Read the model definition and answer for the solid it produces. Units are mm, in the model's axes. Coordinates: 2 decimals unless noted, no trailing zeros. Order: outer loops, then holes, each group sorted by start corner. A loop starts at its lowest first (then second) coordinate and runs counter-clockwise, first axis right, second up.
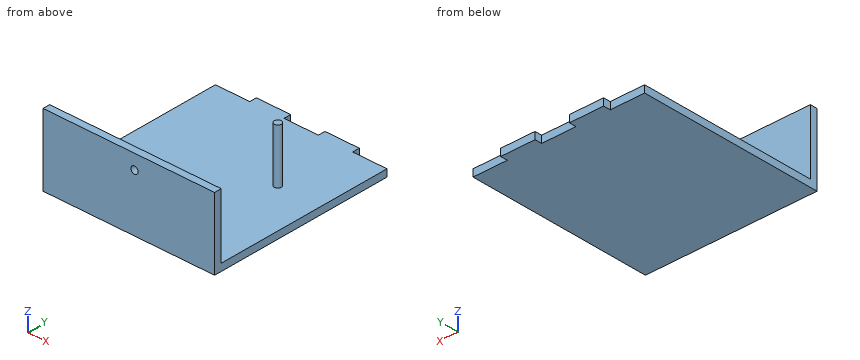
Autodesk Inventor part; units mm, degrees
ref_plane "YZ Plane" through (0, 0, 0) normal (1, 0, 0) x (0, 1, 0)
ref_plane "XZ Plane" through (0, 0, 0) normal (0, 1, 0) x (-1, 0, 0)
ref_plane "XY Plane" through (0, 0, 0) normal (0, 0, 1) x (1, 0, 0)
sketch "Sketch1" plane through (0, 0, 0) normal (0, 0, 1) x (1, 0, 0)
  line L0 (0, 0) -> (120, 0)
  line L1 (120, 0) -> (120, 135)
  line L2 (120, 135) -> (0, 135)
  line L3 (0, 135) -> (0, 0)
  dimension "d0" = 120
  dimension "d1" = 135
extrude "Extrusion1" add sketch "Sketch1" along normal blind 5
sketch "Sketch2" plane through (0, 0, 5) normal (0, 0, 1) x (1, 0, 0)
  line L0 (0, 0) -> (120, 0)
  line L1 (0, 0) -> (120, 0)
  line L2 (120, 0) -> (120, 5)
  line L3 (120, 5) -> (0, 5)
  line L4 (0, 5) -> (0, 0)
  dimension "d4" = 120
  dimension "d5" = 5
extrude "Extrusion2" add sketch "Sketch2" along normal blind 45
sketch "Sketch3" plane through (0, 0, 5) normal (0, 0, 1) x (1, 0, 0)
  line L0 (120, 135) -> (0, 135)
  line L1 (0, 135) -> (24, 135)
  line L2 (24, 135) -> (24, 130)
  line L3 (24, 130) -> (0, 130)
  line L4 (0, 130) -> (0, 135)
  line L5 (120, 135) -> (96, 135)
  line L6 (96, 135) -> (96, 130)
  line L7 (96, 130) -> (120, 130)
  line L8 (120, 130) -> (120, 135)
  line L9 (48, 135) -> (72, 135)
  line L10 (72, 135) -> (72, 130)
  line L11 (72, 130) -> (48, 130)
  line L12 (48, 130) -> (48, 135)
  point P0 (0, 0)
  dimension "d8" = 24
  dimension "d9" = 5
  dimension "d10" = 24
  dimension "d11" = 5
  dimension "d12" = 24
  dimension "d13" = 24
extrude "Extrusion3" cut sketch "Sketch3" against normal blind 45
sketch "Sketch4" plane through (0, 0, 5) normal (0, 0, 1) x (1, 0, 0)
  line L0 (1.8933, 18.6085) -> (59.744, 18.6085) construction
  line L1 (59.744, 18.6085) -> (59.744, 5.8096) construction
  line L2 (59.744, 5.8096) -> (1.8933, 5.8096) construction
  line L3 (1.8933, 5.8096) -> (1.8933, 18.6085) construction
  point P0 (0, 0)
sketch "Sketch5" plane through (0, 0, 0) normal (0, -1, 0) x (1, 0, 0)
  line L0 (1.2536, 49.5181) -> (91.5145, 49.5181) construction
  line L1 (91.5145, 49.5181) -> (91.5145, 35.1014) construction
  line L2 (91.5145, 35.1014) -> (1.2536, 35.1014) construction
  line L3 (1.2536, 35.1014) -> (1.2536, 49.5181) construction
  point P0 (0, 0)
sketch "Sketch6" plane through (0, 5, 5) normal (0, 1, 0) x (1, 0, 0)
  line L0 (39.1274, -43.5353) -> (-30.0492, -43.5353) construction
  line L1 (-30.0492, -43.5353) -> (-30.0492, -68.4744) construction
  line L2 (-30.0492, -68.4744) -> (39.1274, -68.4744) construction
  line L3 (39.1274, -68.4744) -> (39.1274, -43.5353) construction
  point P0 (0, 5)
sketch "Sketch7" plane through (0, 0, 0) normal (0, 0, -1) x (-1, 0, 0)
  line L0 (-119.0942, 8.7754) -> (-47.9511, 8.7754) construction
  line L1 (-47.9511, 8.7754) -> (-47.9511, -14.4167) construction
  line L2 (-47.9511, -14.4167) -> (-119.0942, -14.4167) construction
  line L3 (-119.0942, -14.4167) -> (-119.0942, 8.7754) construction
  point P0 (0, 0)
sketch "Sketch8" plane through (0, 0, 0) normal (0, -1, 0) x (1, 0, 0)
  point P0 (0, 0)
sketch "Sketch9" plane through (0, 0, 0) normal (0, -1, 0) x (1, 0, 0)
  line L0 (120, 0) -> (120, 5)
  line L1 (120, 0) -> (120, 39.815)
  line L2 (120, 39.815) -> (64, 39.815)
  circle A0 centre (64, 39.815) radius 2.5
  point P0 (0, 0)
  dimension "d18" = 39.815
  dimension "d19" = 56
  dimension "d20" = 5
extrude "Extrusion4" cut sketch "Sketch9" against normal blind 10
sketch "Sketch10" plane through (0, 0, 5) normal (0, 0, 1) x (1, 0, 0)
  point P0 (0, 0)
sketch "Sketch11" plane through (0, 0, 5) normal (0, 0, 1) x (1, 0, 0)
  line L0 (120, 5) -> (120, 130)
  line L1 (120, 5) -> (90, 5)
  line L2 (120, 5) -> (0, 5)
  line L3 (90, 5) -> (90, 80)
  circle A0 centre (90, 80) radius 2.5
  point P0 (0, 0)
  dimension "d23" = 30
  dimension "d24" = 75
  dimension "d25" = 5
extrude "Extrusion5" add sketch "Sketch11" along normal blind 38.1
properties part number "WormGearMount"
1) Flat-ended cylindrical pins translate along their axes: pin 1 Ø5 at (x, z) = (97.5, 36.5) entering from +Y; pin 2 Ø5.5 at (x, z) = (9, 3.5) entering from +Y; pin 3 Ø5.5 at (x, y) = (89, 80) entering from +Z; pin 4 Ø6 at (y, z) = (86.5, 30) entering from +X. Find the tip coordinate at first contact, or state that the pin passes through.
A:
pin 1: stops at y = 5
pin 2: stops at y = 130
pin 3: stops at z = 43.1
pin 4: passes through
2) A cutting plane is placed at D-D, the plane x = 109.5. Determine the outline of the cut face in (y, z), and give its area (3 significant figures).
A:
outline: (0, 0) - (130, 0) - (130, 5) - (5, 5) - (5, 50) - (0, 50) - close
area: 875 mm2
3) A cutting plane is placed at B-B, the plane y = 80. Determine the outline of the cut face in (x, z).
A:
outline: (0, 0) - (120, 0) - (120, 5) - (92.5, 5) - (92.5, 43.1) - (87.5, 43.1) - (87.5, 5) - (0, 5) - close
4) A cutting plane is placed at C-C, the plane z = 18.5. Determine the outline of the cut face in (x, y).
A:
outline: (0, 0) - (120, 0) - (120, 5) - (0, 5) - close; circle Ø5 at (90, 80)
5) A cutting plane is placed at A-A, the plane x = 64. Determine the outline of the cut face in (y, z) (3 decimals).
A:
outline: (0, 0) - (130, 0) - (130, 5) - (5, 5) - (5, 37.315) - (0, 37.315) - close; (0, 42.315) - (5, 42.315) - (5, 50) - (0, 50) - close
6) Straight lines are drawn through the part: line 1 (Z direction, x = 64, y = 1.6) (3 decimals); line 2 (Y direction, x = 50, z = 32). For each, find the intervals that lie inside material, in ascending order.
A:
line 1: z = 0 to 37.315, 42.315 to 50
line 2: y = 0 to 5
